Design review of the part built by this model. Coordinates are the model's own, in mm. A direction names the side the tool comes from. Round coordinates to 2 decimals unless told otherwise and drop trailing zeros. One line per item, written item: value. Start each with the question number.
Item 1: Mouldability with a two-part tool opening along Z and no side actions: class faces 3 (the flat face through (3, 0, -3)), 4 (the flat face through (2, -3.7, -2)), 5 (the cylindrical face through (3.29, -1.73, 5.17)), 6 (the flat face through (-3.575, -2, 0)) as released by +Z, released by -Z, zero draft, split by the parting line, or undercut.
Item 2: For faces 1 (the flat face through (-1.76, -1.82, 3.11)), 2 (the flat face through (0, -7, 0)), list the 3-axis set-ups (+Z, -Z, +X, -X, +Y, -Y) from which the entire face can be reached by the end or side of a thin tool; tool diameter is ignored.
Item 3: Clearance check with flat-ended pins moving along their axes: pin 1 (2 mm diameter, centred on x = 3.5, y = -4, fed in from +Z); pin 2 (2 mm diameter, centred on x = -2.5, z = -1, fed in from +Y); pin 3 (2 mm diameter, centred on y = -6, z = -1.5, fed in from +X). State where each tip first meets the part, or that it passes through.
Item 4: For line 1 along Y through (x, z) = (1.25, -0.75); line 2 along Z through (x, y) = (0.75, -2.5); line 3 along Z through (x, y) = (0, -5.1), list the stretches that pass through material, from the lowest coordinate up.
from build123d import *

# Parameters (mm, degrees)
F0_R     = 6.128054
F0_R_2   = 2.25
F1_DEPTH = 7
F2_DEPTH = 5.5
F3_DEPTH = 3.7
F4_R     = 3.5


with BuildPart() as f1:
    # F0 (on Front) → F1 (new body)
    with BuildSketch(Plane.XZ):
        Circle(F0_R)
        Polygon((3.575, 2.064027), (3.575, -2.064027), (0, -4.128054), (-3.575, -2.064027), (-3.575, 2.064027), (0, 4.128054), align=None, mode=Mode.SUBTRACT)
        Polygon((0, -4.128054), (3.575, -2.064027), (3.575, 2.064027), (0, 4.128054), (-3.575, 2.064027), (-3.575, -2.064027), align=None)
        Circle(F0_R_2, mode=Mode.SUBTRACT)
        Circle(F0_R_2)
    extrude(amount=F1_DEPTH)

    # F0 (on Front) → F2 (cut)
    with BuildSketch(Plane.XZ):
        Circle(F0_R_2)
    extrude(amount=F2_DEPTH, mode=Mode.SUBTRACT)

    # F0 (on Front) → F3 (cut)
    with BuildSketch(Plane.XZ):
        Polygon((0, -4.128054), (3.575, -2.064027), (3.575, 2.064027), (0, 4.128054), (-3.575, 2.064027), (-3.575, -2.064027), align=None)
        Circle(F0_R_2, mode=Mode.SUBTRACT)
    extrude(amount=F3_DEPTH, mode=Mode.SUBTRACT)

    # F4
    f4_edges = [f1.edges().sort_by_distance(p)[0] for p in [
        (-6.128054, -7, 0),
    ]]
    fillet(f4_edges, radius=F4_R)


solid = f1.part
A:
1. face 3: zero draft
1. face 4: undercut
1. face 5: split by the parting line
1. face 6: undercut
2. face 1: +Y
2. face 2: +Z, -Z, +X, -X, -Y
3. pin 1: z = 5.57
3. pin 2: y = -3.7
3. pin 3: x = 5.64
4. line 1: -7 to -5.5
4. line 2: -6.08 to -3.7, 3.7 to 6.08
4. line 3: -5.74 to -2.25, 2.25 to 5.74
